```python
from build123d import *

# Parameters (mm, degrees)
F0_R     = 20
F0_R_2   = 1.7
F1_DEPTH = 2
F2_R     = 20
F2_R_2   = 15
F2_R_3   = 7.5
F2_R_4   = 1.7
F3_DEPTH = 5
F4_W     = 10
F4_H     = 10
F5_DEPTH = 5
F6_R     = 1.7
F7_DEPTH = 2.6


with BuildPart() as f1:
    # F0 (on Top) → F1 (new body)
    with BuildSketch(Plane.XY):
        Circle(F0_R)
        Circle(F0_R_2, mode=Mode.SUBTRACT)
    extrude(amount=F1_DEPTH)

    # F2 (on face) → F3 (join)
    with BuildSketch(Plane.XY.offset(2)):
        Circle(F2_R)
        Circle(F2_R_2, mode=Mode.SUBTRACT)
        Circle(F2_R_3)
        Circle(F2_R_4, mode=Mode.SUBTRACT)
    extrude(amount=F3_DEPTH)

    # F4 (on face) → F5 (cut, through all)
    with BuildSketch(Plane.XY.offset(7)):
        with Locations((-18, 0)):
            Rectangle(F4_W, F4_H)
        Polygon((-12.7279220614, -5.6568542495), (-19.7989898732, -12.7279220614), (-12.7279220614, -19.7989898732), (-5.6568542495, -12.7279220614), align=None)
        with Locations((0, -18)):
            Rectangle(F4_W, F4_H)
        Polygon((5.6568542495, -12.7279220614), (12.7279220614, -19.7989898732), (19.7989898732, -12.7279220614), (12.7279220614, -5.6568542495), align=None)
        with Locations((18, 0)):
            Rectangle(F4_W, F4_H)
        Polygon((12.7279220614, 5.6568542495), (19.7989898732, 12.7279220614), (12.7279220614, 19.7989898732), (5.6568542495, 12.7279220614), align=None)
        with Locations((0, 18)):
            Rectangle(F4_W, F4_H)
        Polygon((-5.6568542495, 12.7279220614), (-12.7279220614, 19.7989898732), (-19.7989898732, 12.7279220614), (-12.7279220614, 5.6568542495), align=None)
    extrude(amount=-F5_DEPTH, mode=Mode.SUBTRACT)

    # F6 (on face) → F7 (cut)
    with BuildSketch(Plane(origin=(0, 0, 0), x_dir=(1, 0, 0), z_dir=(0, 0, -1))):
        Polygon((2.95, -1.7031832941), (2.95, 1.7031832941), (0, 3.4063665882), (-2.95, 1.7031832941), (-2.95, -1.7031832941), (0, -3.4063665882), align=None)
        Circle(F6_R, mode=Mode.SUBTRACT)
    extrude(amount=-F7_DEPTH, mode=Mode.SUBTRACT)


solid = f1.part
```
Model file for the job. Use its own axes, mm. A direction names the side the tool comes from. Round coordinates to 2 decimals unless told otherwise and drop trailing zeros. Order: outer loops, then holes, each group sorted by start corner. A loop starts at its lowest first (then second) coordinate and runs counter-clockwise, first axis right, second up. Notation, with made-up numbers: (17, -5.75) -> (38, -5.75) arc R28 cw to (38, 19.25) -> close; hole circle Ø8 at (-7, 76.5). An arc over 180 degrees is marked (long way). Use one line per item in the form item = value.
Item 1: Cut at D-D, the plane x = -3.5. Write the cut outline in (y, z), and give its area (3 significant figures).
Returned:
outline = (-19.69, 0) -> (19.69, 0) -> (19.69, 2) -> (6.63, 2) -> (6.63, 7) -> (-6.63, 7) -> (-6.63, 2) -> (-19.69, 2) -> close
area = 145 mm^2
Item 2: Pull direction Y, two halves, no side cores. Call faces 1 (the face through (-16, 7, 7)), 2 (the face through (18.475, -7.66, 2.673)), 3 (the face through (17, 5, 5)): released by +Y, released by -Y, zero draft, split by the parting line, or undercut.
Returned:
face_1 = zero draft
face_2 = split by the parting line
face_3 = undercut
Item 3: Cut at C-C, the plane z = 0.5. Write the cut outline in (x, y), and give its area (3 significant figures).
Returned:
outline = circle Ø40 at (0, 0); hole (-2.95, -1.7) -> (0, -3.41) -> (2.95, -1.7) -> (2.95, 1.7) -> (0, 3.41) -> (-2.95, 1.7) -> close
area = 1,230 mm^2
Item 4: Cut at A-A, the plane y = 0. Write the cut outline in (x, z).
Returned:
outline = (-20, 0) -> (-2.95, 0) -> (-2.95, 2.6) -> (-1.7, 2.6) -> (-1.7, 7) -> (-7.5, 7) -> (-7.5, 2) -> (-20, 2) -> close; (1.7, 2.6) -> (2.95, 2.6) -> (2.95, 0) -> (20, 0) -> (20, 2) -> (7.5, 2) -> (7.5, 7) -> (1.7, 7) -> close
Item 5: Tool access for faces 4 (the face through (1.45, 2.57, 1.28)), 5 (the face through (-5.73, 13.862, 4.465)), 6 (the face through (17, -5, 5)): list every direction of +Z, -Z, +X, -X, +Y, -Y with a clear straight run to the whole face (end or side of a thin tool).
Returned:
face_4 = -Z
face_5 = +Z
face_6 = +Z, +X
Item 6: Drill centre lines: line 1 (Y direction, x = 0, z = 5.65); line 2 (Z direction, x = -2.5, y = -9.5); line 3 (Y direction, x = 8, z = 6). Where is each one in solid material? Low to high.
Returned:
line_1 = -7.5 to -1.7, 1.7 to 7.5
line_2 = 0 to 2
line_3 = -18.33 to -15.07, 15.07 to 18.33
Item 7: Cut at B-B, the plane z = 3.5. Give the number of separate pieces and of enclosed holes in the cut face, and give its area (3 significant figures).
Returned:
separate_pieces = 9
enclosed_holes = 1
area = 312 mm^2
Item 8: Flat gauge pins, fed straight in: pin 1 Ø4 at (x, z) = (11, 4) entering from -Y; pin 2 Ø2 at (x, y) = (0, 0) entering from -Z; pin 3 Ø4 at (x, y) = (13.5, -14) entering from +Z; pin 4 Ø1 at (y, z) = (-15.5, 6) entering from +X. Where does each tip first touch, or does it go through?
Returned:
pin_1 = -17.86
pin_2 = through
pin_3 = 2
pin_4 = 8.93
